from build123d import *

# Parameters (mm, degrees)
SKETCH1_W           = 33.3
SKETCH1_H           = 33.3
SKETCH1_W_2         = 22.8
SKETCH1_H_2         = 22.8
BOSS_EXTRUDE1_DEPTH = 1.5
SKETCH1_3_W         = 22.8
SKETCH1_3_H         = 22.8
BOSS_EXTRUDE2_DEPTH = 5
FILLET1_R           = 4.5
CHAMFER1_SIZE       = 1


with BuildPart() as part:
    # Sketch1 → Boss-Extrude1 (new body)
    # profile 1 of 2: a face of its own
    with BuildSketch(Plane(origin=(0, 0, 0), x_dir=(1, 0, 0), z_dir=(0, 1, 0))):
        Rectangle(SKETCH1_W, SKETCH1_H)
        Rectangle(SKETCH1_W_2, SKETCH1_H_2, mode=Mode.SUBTRACT)
    # profile 2 of 2: a face of its own
    with BuildSketch(Plane(origin=(0, 0, 0), x_dir=(1, 0, 0), z_dir=(0, 1, 0))):
        Rectangle(SKETCH1_W_2, SKETCH1_H_2)
    extrude(amount=BOSS_EXTRUDE1_DEPTH)

    # Sketch1_3 → Boss-Extrude2 (add)
    with BuildSketch(Plane(origin=(0, 0, 0), x_dir=(1, 0, 0), z_dir=(0, 1, 0))):
        Rectangle(SKETCH1_3_W, SKETCH1_3_H)
    extrude(amount=BOSS_EXTRUDE2_DEPTH)

    # Fillet1
    fillet1_edges = [part.edges().sort_by_distance(p)[0] for p in [
        (-11.4, 3.25, 11.4),
        (11.4, 3.25, 11.4),
        (11.4, 3.25, -11.4),
        (-11.4, 3.25, -11.4),
        (-16.65, 0.75, 16.65),
        (-16.65, 0.75, -16.65),
        (16.65, 0.75, -16.65),
        (16.65, 0.75, 16.65),
    ]]
    fillet(fillet1_edges, radius=FILLET1_R)

    # Chamfer1
    chamfer1_edges = [part.edges().sort_by_distance(p)[0] for p in [
        (16.65, 1.5, 0),
        (0, 1.5, 16.65),
        (0, 1.5, -16.65),
        (-16.65, 1.5, 0),
        (-15.331980515, 1.5, 15.331980515),
        (-15.331980515, 1.5, -15.331980515),
        (15.331980515, 1.5, -15.331980515),
        (15.331980515, 1.5, 15.331980515),
    ]]
    chamfer(chamfer1_edges, length=CHAMFER1_SIZE)


solid = part.part
Could you check a few things on this model? Use its own coordinates, in mm. A direction names the side the tool comes from. Give positions to 0.01 mm unless a question says otherwise; leave off trailing zeros. Order: outer loops, then holes, each group sorted by start corner. A loop starts at its lowest first (then second) coordinate and runs counter-clockwise, first axis right, second up.
1. I need wall thicknesses on L1, parallel to Y at x = -5, z = -13.5; L2, parallel to Z at x = -5, y = 3.2. Which ranges of each line are inside material? Lowest first, please.
Answers below:
L1: y = 0 to 1.5
L2: z = -11.4 to 11.4
2. Which directions (+Z, -Z, +X, -X, +Y, -Y) give clear straight access to the entire face, cutting with the end or side of a thin tool? Please do faces 1 (the cylindrical face through (-10.117, 3.274, 10.047)), 2 (the flat face through (0, 3, 11.4)), 3 (the cylindrical face through (10.047, 3.274, 10.117)).
Answers below:
face 1: +Z, -X, +Y
face 2: +Z, +X, -X, +Y
face 3: +Z, +X, +Y
3. Suppose I cut it at D-D (y = 3.9). Write out the boundary of the cut face in (x, z), plus the area to 3 significant figures.
Answers below:
outline: (-11.4, -6.9) arc R4.5 ccw to (-6.9, -11.4) - (6.9, -11.4) arc R4.5 ccw to (11.4, -6.9) - (11.4, 6.9) arc R4.5 ccw to (6.9, 11.4) - (-6.9, 11.4) arc R4.5 ccw to (-11.4, 6.9) - close
area: 502 mm2
4. Suppose I cut it at C-C (x = -4.5). Write out the boundary of the cut face in (y, z), plus the area to 3 significant figures.
Answers below:
outline: (0, -16.65) - (0.5, -16.65) - (1.5, -15.65) - (1.5, -11.4) - (5, -11.4) - (5, 11.4) - (1.5, 11.4) - (1.5, 15.65) - (0.5, 16.65) - (0, 16.65) - close
area: 129 mm2
5. Suppose I cut it at A-A (z = -5.5). Write out the boundary of the cut face in (x, y).
Answers below:
outline: (-16.65, 0) - (16.65, 0) - (16.65, 0.5) - (15.65, 1.5) - (11.4, 1.5) - (11.4, 5) - (-11.4, 5) - (-11.4, 1.5) - (-15.65, 1.5) - (-16.65, 0.5) - close
6. For pin 1 (1.5 mm diameter, centred on y = 1.5, z = -1.5, fed in from -X); pin 2 (1 mm diameter, centred on x = 0.5, y = 2.5, fed in from +Z); pin 3 (3 mm diameter, centred on x = 7, y = 4.5, fed in from -Z), each with a flat end and sliding along its axis, tell me the tip position at first contact or that it passes through.
Answers below:
pin 1: stops at x = -16.4
pin 2: stops at z = 11.4
pin 3: stops at z = -11.4
7. Suppose I cut it at B-B (y = 1.05). Write out the boundary of the cut face in (x, z), plus the area to 3 significant figures.
Answers below:
outline: (-16.1, -12.15) arc R3.95 ccw to (-12.15, -16.1) - (12.15, -16.1) arc R3.95 ccw to (16.1, -12.15) - (16.1, 12.15) arc R3.95 ccw to (12.15, 16.1) - (-12.15, 16.1) arc R3.95 ccw to (-16.1, 12.15) - close
area: 1,020 mm2
